Autodesk Inventor part; units mm, degrees
ref_plane "YZ Plane" through (0, 0, 0) normal (1, 0, 0) x (0, 1, 0)
ref_plane "XZ Plane" through (0, 0, 0) normal (0, 1, 0) x (-1, 0, 0)
ref_plane "XY Plane" through (0, 0, 0) normal (0, 0, 1) x (1, 0, 0)
sketch "Szkic1" plane through (0, 0, 0) normal (0, 1, 0) x (-1, 0, 0)
  line L0 (25, 20) -> (5, 20)
  line L1 (5, 20) -> (5, 0)
  line L2 (5, 0) -> (25, 0)
  line L3 (25, 0) -> (25, 20)
  line L4 (-5, 20) -> (-25, 20)
  line L5 (-25, 20) -> (-25, 0)
  line L6 (-25, 0) -> (-5, 0)
  line L7 (-5, 0) -> (-5, 20)
  line L8 (25, 0) -> (-25, 0)
  line L9 (-25, 0) -> (-25, 30)
  line L10 (-25, 30) -> (25, 30)
  line L11 (25, 30) -> (25, 0)
  point P0 (0, 0)
  point P1 (-15, 20)
  point P2 (15, 20)
  point P3 (15, 0)
  point P4 (-5, 0)
  point P5 (5, 0)
  dimension "d0" = 20
  dimension "d1" = 20
  dimension "d2" = 20
  dimension "d3" = 20
  dimension "d4" = 50
  dimension "d5" = 25
  dimension "d6" = 10
extrude "Wyciągnięcie proste1" add sketch "Szkic1" along normal blind 20 contours L0 L1 L8 L7 L4 L9 L10 L11
sketch "Szkic2" plane through (5, 0, 0) normal (0, 0, -1) x (-1, 0, 0)
  circle A0 centre (5, 10) radius 3.25
  circle A1 centre (20, 10) radius 2.25
  circle A2 centre (-10, 10) radius 2.25
  line L0 (0, 0) -> (0, 20)
  line L1 (0, 0) -> (10, 0)
  line L2 (-20, 0) -> (-20, 20)
  line L3 (-20, 0) -> (0, 0)
  line L4 (30, 0) -> (30, 20)
  circle A3 centre (-10, 10) radius 4
  circle A4 centre (20, 10) radius 4
  line L5 (1.8246, 15.5) -> (8.1754, 15.5)
  line L6 (8.1754, 15.5) -> (11.3509, 10)
  line L7 (11.3509, 10) -> (8.1754, 4.5)
  line L8 (8.1754, 4.5) -> (1.8246, 4.5)
  line L9 (1.8246, 4.5) -> (-1.3509, 10)
  line L10 (-1.3509, 10) -> (1.8246, 15.5)
  point P0 (5, 0)
  dimension "d9" = 6.5
  dimension "d10" = 5
  dimension "d11" = 10
  dimension "d12" = 10
  dimension "d13" = 10
  dimension "d14" = 10
  dimension "d15" = 4.5
  dimension "d16" = 4.5
  dimension "d20" = 8
  dimension "d21" = 8
  dimension "d25" = 11
extrude "Wyciągnięcie proste2" cut sketch "Szkic2" against normal through all contours A0 | A1 | A2
extrude "Wyciągnięcie proste3" cut sketch "Szkic2" along normal blind 5 from surface at -30 contours A0 | L9 L10 L0 | L0 L10 L5 L6 L7 L8 L9
fillet "Zaokrąglenie1" radius 6 2 edges at (25, 10, 30) (-25, 10, 30)
extrude "Wyciągnięcie proste4" cut sketch "Szkic2" along normal blind 1 from surface at -30 contours A1 | A2 | A3 | A4
properties part number "Z_item_mount" material "Tworzywo sztuczne ABS"
Here's how the part is built. I have some questions about the finished solid (model axes, mm). A direction names the side the tool comes from. Give positions to 0.01 mm unless a question says otherwise; leave off trailing zeros. Order: outer loops, then holes, each group sorted by start corner. A loop starts at its lowest first (then second) coordinate and runs counter-clockwise, first axis right, second up. Notation, with made-up numbers: (30, -30.75) - (54, -30.75) arc R32 ccw to (54, 1.25) - close; hole circle Ø4 at (-16.5, 61). An arc over 180 degrees is marked (long way). Answer as a JSON object with one key per item and string values. Group by question number.
Item 1: If we mould it in two halves opening along X, with no side actions, what happens to faces 1 (the flat face through (-3.4, 9.9, 0)), 2 (the cylindrical face through (0.423, 13.222, 12.325)), 3 (the flat face through (-25, 10, 22))? For each: pulls with the +X half, pulls with the -X half, needs draft (parallel to the pull), parting line crosses it, or undercut.
Item 2: Please list where these lines run through material, in increasing order: probe 1 along Y at (x, z) = (15, 29.7); probe 2 along Z at (x, y) = (-11.5, 3.5); probe 3 along X at (y, z) = (3, 6.5).
Item 3: For P1, Ø10, axis at y = 12.5, z = 8, coming from the +X side; P2, Ø2.5, axis at x = -16.5, y = 11, coming from the +Z side; P3, Ø6, axis at y = 13, z = 7.5, coming from the -X side, each with a flat end and sliding along its axis, tell me the tip position at first contact or that it passes through.
Item 4: If we section it at C-C on z = 17: Please give me the cut outline in (x, y), and give its area (3 significant figures).
Item 5: If we section it at D-D on x = 0: Please give me the cut outline in (y, z), and give its area (4 significant figures).
Item 6: If we section it at B-B on y = 11.5: Give the number of separate pieces and of enclosed holes in the cut face, and give its area (3 significant figures).
Item 7: If we section it at A-A on x = -15: Please give me the cut outline in (y, z), and give its area (4 significant figures).
Item 8: Which directions (+Z, -Z, +X, -X, +Y, -Y) give clear straight access to the entire face, cutting with the end or side of a thin tool? Please do faces 4 (the cylindrical face through (23.196, 10.14, 28.289)), 5 (the flat face through (-5, 10, 10)), 6 (the cylindrical face through (-11.8, 12.4, 29.5)).
Result set:
{
 "1": {"face 1": "needs draft", "face 2": "undercut", "face 3": "pulls with the -X half"},
 "2": {"probe 1": "0 to 6, 14 to 20", "probe 2": "20 to 30", "probe 3": "-5 to 5"},
 "3": {"P1": "x = 5", "P2": "z = 29", "P3": "x = -5"},
 "4": {"outline": "(-5, 0) - (5, 0) - (5, 20) - (-5, 20) - close; hole circle Ø6.5 at (0, 10)", "area": "167 mm²"},
 "5": {"outline": "(0, 0) - (6.75, 0) - (6.75, 25) - (4.5, 25) - (4.5, 30) - (0, 30) - close; (13.25, 0) - (20, 0) - (20, 30) - (15.5, 30) - (15.5, 25) - (13.25, 25) - close", "area": "382.5 mm²"},
 "6": {"separate pieces": "4", "enclosed holes": "0", "area": "410 mm²"},
 "7": {"outline": "(0, 20) - (7.75, 20) - (7.75, 29) - (6, 29) - (6, 30) - (0, 30) - close; (12.25, 20) - (20, 20) - (20, 30) - (14, 30) - (14, 29) - (12.25, 29) - close", "area": "151.5 mm²"},
 "8": {"face 4": "+Z, +X, +Y, -Y", "face 5": "-Z, -X, +Y, -Y", "face 6": "+Z"}
}
